The listing builds one solid part. Answer for the finished solid, in the listing's coordinates (mm). A direction names the side the tool comes from. Give positions to 0.01 mm unless a question says otherwise; leave off trailing zeros. Loops run counter-clockwise (first coordinate to the right, second up) from the corner with the lowest first, then second, coordinate; pieces in that order, holes last. Notation, with made-up numbers: (25.5, 67) - (59.5, 67) arc R34 ccw to (59.5, 100) - close; hole circle Ø2 at (77, -17.5). An arc over 180 degrees is marked (long way). Write item = value, one per line. Start each with the question number.
1) Consider probe 1 along X at (y, z) = (-6.5, -1.75); probe 2 along Y at (x, z) = (1.85, 0); probe 3 along Z at (x, y) = (2.5, -0.5). Determine where each line is inside the solid, lowest interval first.
2) The part is cut by section A-A on x = 3.75. Write down the section's boundary in (y, z).
3) Flat-ended cylindrical pins translate along their axes: P1, Ø4, axis at y = 0, z = 0, coming from the +X side; P2, Ø1.5, axis at x = -0.5, y = 2, coming from the -Z side; P3, Ø4, axis at x = 3, y = 3.5, coming from the +Z side; P4, Ø1.5, axis at x = 0, z = -5.5, coming from the +Y side. Find the tip coordinate at first contact, or state that the pin passes through.
4) Which of the six approach directions +Z, -Z, +X, -X, +Y, -Y give full straight-line access (tool end or side, diameter ignored) to faces 1 (the flat face through (4.25, 2, 0)), 2 (the flat face through (-3.25, 6, -2))?
from build123d import *

# Parameters (mm, degrees)
CHAMFER1_SIZE = 0.2


with BuildPart() as part:
    # Sketch1 → Revolve1 (revolve)
    with BuildSketch(Plane.XY, mode=Mode.PRIVATE) as revolve1_sk:
        Polygon((-4.25, 1.5), (-4.25, 2.4), (-4.05, 2.6), (-4.25, 2.8), (-4.25, 9), (-3.25, 9), (-3.25, 6), (0, 6), (0, 1.5), align=None)
    revolve(revolve1_sk.sketch.rotate(Axis((0, 0, 0), (-1, 0, 0)), 90), axis=Axis((0, 0, 0), (-1, 0, 0)))

    # Mirror1: part across plane


with BuildPart() as part_1:
    add(part.part)
    add(part.part.mirror(Plane(origin=(0, 6, 0), x_dir=(0, 0, 1), z_dir=(1, 0, 0))))

    # Chamfer1
    chamfer1_edges = [part_1.edges().sort_by_distance(p)[0] for p in [
        (-4.25, 0, 9),
        (4.25, 0, 9),
        (3.25, 0, 9),
        (-3.25, 0, 9),
    ]]
    chamfer(chamfer1_edges, length=CHAMFER1_SIZE)


solid = part_1.part
Answer below:
q1.probe_1 = -4.25 to -3.25, 3.25 to 4.25
q1.probe_2 = -6 to -1.5, 1.5 to 6
q1.probe_3 = -5.98 to -1.41, 1.41 to 5.98
q2.outline = circle Ø18 at (0, 0); hole circle Ø3 at (0, 0)
q3.P1 = 4.25
q3.P2 = -5.87
q3.P3 = 8.87
q3.P4 = 3.67
q4.face_1 = +Z, -Z, +X, +Y, -Y
q4.face_2 = none
